```python
from build123d import *

# Parameters (mm, degrees)
BOSS_EXTRUDE1_DEPTH = 107.95


with BuildPart() as part:
    # Sketch1 → Boss-Extrude1 (new body)
    with BuildSketch(Plane(origin=(0, 0, 0), x_dir=(0, 0, -1), z_dir=(1, 0, 0))):
        Polygon((7.332348419, 0), (3.666174209, 6.35), (-3.666174209, 6.35), (-7.332348419, 0), (-3.666174209, -6.35), (3.666174209, -6.35), align=None)
        Polygon((2.886751346, 0), (1.443375673, 2.5), (-1.443375673, 2.5), (-2.886751346, 0), (-1.443375673, -2.5), (1.443375673, -2.5), align=None, mode=Mode.SUBTRACT)
    extrude(amount=BOSS_EXTRUDE1_DEPTH)


solid = part.part
```
The model under review builds one solid part; all positions refer to its coordinate system, in mm. A direction names the side the tool comes from. Round coordinates to 2 decimals unless told otherwise and drop trailing zeros. Loops run counter-clockwise (first coordinate to the right, second up) from the corner with the lowest first, then second, coordinate; pieces in that order, holes last.
1) The part is to be moulded in two halves that separate along Z. For faces 1 (the face through (53.219, 3.219, 5.474)), 2 (the face through (53.219, -1.267, -2.155)), 3 (the face through (53, 6.35, 0)), 4 (the face through (53.219, 1.267, 2.155)), say which applies: pulls with the +Z half, pulls with the -Z half, needs draft (parallel to the pull), parting line crosses it, or undercut.
Values follow:
face 1: pulls with the +Z half
face 2: undercut
face 3: needs draft
face 4: undercut
2) Tool access review of faces 5 (the face through (53.219, 3.131, -5.525)), 6 (the face through (53, -2.5, 0)): name each direction out of +Z, -Z, +X, -X, +Y, -Y from which nothing blocks a thin tool from reaching the whole face with its end or side.
Values follow:
face 5: -Z, +X, -X, +Y
face 6: +X, -X
3) Consider section B-B on y = -1.25. State the section outline as (x, z) points, then the cut area to 3 significant figures.
Values follow:
outline: (0, -6.61) - (107.95, -6.61) - (107.95, -2.17) - (0, -2.17) - close; (0, 2.17) - (107.95, 2.17) - (107.95, 6.61) - (0, 6.61) - close
area: 960 mm2
4) Wall thickness on line 1 along Y through (x, z) = (23.5, 0.5); line 2 along Y through (x, z) = (92, -1.75); line 3 along Z through (x, y) = (79, 0.25): over which ranges is each line inside the solid? List them lowest first.
Values follow:
line 1: y = -6.35 to -2.5, 2.5 to 6.35
line 2: y = -6.35 to -1.97, 1.97 to 6.35
line 3: z = -7.19 to -2.74, 2.74 to 7.19
5) Consider section C-C on y = -5.25. State the section outline as (x, z) points.
Values follow:
outline: (0, -4.3) - (107.95, -4.3) - (107.95, 4.3) - (0, 4.3) - close
6) Consider section A-A on x = 78. State the section outline as (y, z) points, then the cut area to 3 significant figures.
Values follow:
outline: (-6.35, -3.67) - (0, -7.33) - (6.35, -3.67) - (6.35, 3.67) - (0, 7.33) - (-6.35, 3.67) - close; hole (-2.5, -1.44) - (0, -2.89) - (2.5, -1.44) - (2.5, 1.44) - (0, 2.89) - (-2.5, 1.44) - close
area: 118 mm2
7) Consider section D-D on z = 5.5. State the section outline as (x, y) points.
Values follow:
outline: (0, -3.17) - (107.95, -3.17) - (107.95, 3.17) - (0, 3.17) - close
